Can you work these out from the model? Positions are in its coordinate system, mm. A direction names the side the tool comes from. Give positions to 0.01 mm unless a question says otherwise; leave off trailing zeros. Loops run counter-clockwise (first coordinate to the right, second up) from the corner with the lowest first, then second, coordinate; pieces in that order, holes last. Notation, with made-up numbers: (43.25, 85) -> (62.25, 85) arc R10 cw to (62.25, 101) -> close; hole circle Ø11 at (-28, 78.5). An arc over 180 degrees is marked (long way). One line per question, with ' | ' between items.
from build123d import *

# Parameters (mm, degrees)
F0_W     = 63.2
F0_H     = 30.7
F1_DEPTH = 9
F2_R     = 4.5
F2_R_2   = 3
F3_DEPTH = 3.5
F4_T     = 1


# Not quite as in the source:
# - a shell that OpenCascade refuses in one call is made with other operations: the cavity is built on its own and cut out


with BuildPart() as f1:
    # F0 (on Front) → F1 (new body)
    with BuildSketch(Plane.XZ):
        with Locations((2.7909118284, 0)):
            Rectangle(F0_W, F0_H)
    extrude(amount=F1_DEPTH)

    # F2 (on face) → F3 (join)
    with BuildSketch(Plane.XZ.offset(9)):
        with Locations((-21.0856401334, 7.675)):
            Circle(F2_R)
        with Locations((-21.0856401334, 7.675)):
            Circle(F2_R_2, mode=Mode.SUBTRACT)
        with Locations((-4.9325362097, 7.675)):
            Circle(F2_R)
        with Locations((-4.9325362097, 7.675)):
            Circle(F2_R_2, mode=Mode.SUBTRACT)
        with Locations((10.5143598666, 7.675)):
            Circle(F2_R)
        with Locations((10.5143598666, 7.675)):
            Circle(F2_R_2, mode=Mode.SUBTRACT)
        with Locations((-4.9325362097, -7.675)):
            Circle(F2_R)
        with Locations((-4.9325362097, -7.675)):
            Circle(F2_R_2, mode=Mode.SUBTRACT)
        with Locations((10.5143598666, -7.675)):
            Circle(F2_R)
        with Locations((10.5143598666, -7.675)):
            Circle(F2_R_2, mode=Mode.SUBTRACT)
        with Locations((-21.0856401334, -7.675)):
            Circle(F2_R)
        with Locations((-21.0856401334, -7.675)):
            Circle(F2_R_2, mode=Mode.SUBTRACT)
        with Locations((26.6674637903, -7.675)):
            Circle(F2_R)
        with Locations((26.6674637903, -7.675)):
            Circle(F2_R_2, mode=Mode.SUBTRACT)
        with Locations((26.6674637903, 7.675)):
            Circle(F2_R)
        with Locations((26.6674637903, 7.675)):
            Circle(F2_R_2, mode=Mode.SUBTRACT)
    extrude(amount=F3_DEPTH)

    # F4: shell of thickness 1, made by hand


with BuildPart() as f4_core1:
    # F4_t2: copy of F1
    add(f1.part)

    # the walls: a layer under each face that stays
    f4_faces = [f4_core1.faces().sort_by_distance(p)[0] for p in [
        (2.7909118284, -4.5, -15.35),
        (-28.8090881716, -4.5, 0),
        (34.3909118284, -4.5, 0),
        (2.7909118284, -9, 0),
        (2.7909118284, -4.5, 15.35),
        (-25.5856401334, -10.75, -7.675),
        (-9.4325362097, -10.75, -7.675),
        (6.0143598666, -10.75, -7.675),
        (22.1674637903, -10.75, -7.675),
        (-25.5856401334, -10.75, 7.675),
        (-9.4325362097, -10.75, 7.675),
        (6.0143598666, -10.75, 7.675),
        (22.1674637903, -10.75, 7.675),
        (-24.0856401334, -12.5, -10.675),
        (-7.9325362097, -12.5, -10.675),
        (7.5143598666, -12.5, -10.675),
        (23.6674637903, -12.5, -10.675),
        (-24.0856401334, -12.5, 4.675),
        (-7.9325362097, -12.5, 4.675),
        (7.5143598666, -12.5, 4.675),
        (23.6674637903, -12.5, 4.675),
        (-24.0856401334, -10.75, -7.675),
        (-7.9325362097, -10.75, -7.675),
        (7.5143598666, -10.75, -7.675),
        (23.6674637903, -10.75, -7.675),
        (-24.0856401334, -10.75, 7.675),
        (-7.9325362097, -10.75, 7.675),
        (7.5143598666, -10.75, 7.675),
        (23.6674637903, -10.75, 7.675),
        (-21.0856401334, -9, -7.675),
        (-4.9325362097, -9, -7.675),
        (10.5143598666, -9, -7.675),
        (26.6674637903, -9, -7.675),
        (-21.0856401334, -9, 7.675),
        (-4.9325362097, -9, 7.675),
        (10.5143598666, -9, 7.675),
        (26.6674637903, -9, 7.675),
    ]]
    thicken(f4_faces, amount=-F4_T, mode=Mode.SUBTRACT)

    # F4_s3 → F4_t4 (revolve, cut)
    with BuildSketch(Plane.XY.offset(-7.675)):
        Polygon((-16.5756401334, -9.01), (-16.5856401334, -8), (-17.5856401334, -8), (-17.5856401334, -9), align=None)
    revolve(axis=Axis((-21.0856401334, -9, -7.675), (0, -1, 0)), mode=Mode.SUBTRACT)

    # F4_s5 → F4_t6 (revolve, cut)
    with BuildSketch(Plane.XY.offset(-7.675)):
        Polygon((-0.4225362097, -9.01), (-0.4325362097, -8), (-1.4325362097, -8), (-1.4325362097, -9), align=None)
    revolve(axis=Axis((-4.9325362097, -9, -7.675), (0, -1, 0)), mode=Mode.SUBTRACT)

    # F4_s7 → F4_t8 (revolve, cut)
    with BuildSketch(Plane.XY.offset(-7.675)):
        Polygon((15.0243598666, -9.01), (15.0143598666, -8), (14.0143598666, -8), (14.0143598666, -9), align=None)
    revolve(axis=Axis((10.5143598666, -9, -7.675), (0, -1, 0)), mode=Mode.SUBTRACT)

    # F4_s9 → F4_t10 (revolve, cut)
    with BuildSketch(Plane.XY.offset(-7.675)):
        Polygon((31.1774637903, -9.01), (31.1674637903, -8), (30.1674637903, -8), (30.1674637903, -9), align=None)
    revolve(axis=Axis((26.6674637903, -9, -7.675), (0, -1, 0)), mode=Mode.SUBTRACT)

    # F4_s11 → F4_t12 (revolve, cut)
    with BuildSketch(Plane.XY.offset(7.675)):
        Polygon((-16.5756401334, -9.01), (-16.5856401334, -8), (-17.5856401334, -8), (-17.5856401334, -9), align=None)
    revolve(axis=Axis((-21.0856401334, -9, 7.675), (0, -1, 0)), mode=Mode.SUBTRACT)

    # F4_s13 → F4_t14 (revolve, cut)
    with BuildSketch(Plane.XY.offset(7.675)):
        Polygon((-0.4225362097, -9.01), (-0.4325362097, -8), (-1.4325362097, -8), (-1.4325362097, -9), align=None)
    revolve(axis=Axis((-4.9325362097, -9, 7.675), (0, -1, 0)), mode=Mode.SUBTRACT)

    # F4_s15 → F4_t16 (revolve, cut)
    with BuildSketch(Plane.XY.offset(7.675)):
        Polygon((15.0243598666, -9.01), (15.0143598666, -8), (14.0143598666, -8), (14.0143598666, -9), align=None)
    revolve(axis=Axis((10.5143598666, -9, 7.675), (0, -1, 0)), mode=Mode.SUBTRACT)

    # F4_s17 → F4_t18 (revolve, cut)
    with BuildSketch(Plane.XY.offset(7.675)):
        Polygon((31.1774637903, -9.01), (31.1674637903, -8), (30.1674637903, -8), (30.1674637903, -9), align=None)
    revolve(axis=Axis((26.6674637903, -9, 7.675), (0, -1, 0)), mode=Mode.SUBTRACT)

    # F4_s19 → F4_t20 (revolve, cut)
    with BuildSketch(Plane.XY.offset(-7.675)):
        Polygon((-18.0956401334, -9.01), (-17.0856401334, -9), (-17.0856401334, -8), (-18.0856401334, -8), align=None)
    revolve(axis=Axis((-21.0856401334, -9, -7.675), (0, -1, 0)), mode=Mode.SUBTRACT)

    # F4_s21 → F4_t22 (revolve, cut)
    with BuildSketch(Plane.XY.offset(-7.675)):
        Polygon((-1.9425362097, -9.01), (-0.9325362097, -9), (-0.9325362097, -8), (-1.9325362097, -8), align=None)
    revolve(axis=Axis((-4.9325362097, -9, -7.675), (0, -1, 0)), mode=Mode.SUBTRACT)

    # F4_s23 → F4_t24 (revolve, cut)
    with BuildSketch(Plane.XY.offset(-7.675)):
        Polygon((13.5043598666, -9.01), (14.5143598666, -9), (14.5143598666, -8), (13.5143598666, -8), align=None)
    revolve(axis=Axis((10.5143598666, -9, -7.675), (0, -1, 0)), mode=Mode.SUBTRACT)

    # F4_s25 → F4_t26 (revolve, cut)
    with BuildSketch(Plane.XY.offset(-7.675)):
        Polygon((29.6574637903, -9.01), (30.6674637903, -9), (30.6674637903, -8), (29.6674637903, -8), align=None)
    revolve(axis=Axis((26.6674637903, -9, -7.675), (0, -1, 0)), mode=Mode.SUBTRACT)

    # F4_s27 → F4_t28 (revolve, cut)
    with BuildSketch(Plane.XY.offset(7.675)):
        Polygon((-18.0956401334, -9.01), (-17.0856401334, -9), (-17.0856401334, -8), (-18.0856401334, -8), align=None)
    revolve(axis=Axis((-21.0856401334, -9, 7.675), (0, -1, 0)), mode=Mode.SUBTRACT)

    # F4_s29 → F4_t30 (revolve, cut)
    with BuildSketch(Plane.XY.offset(7.675)):
        Polygon((-1.9425362097, -9.01), (-0.9325362097, -9), (-0.9325362097, -8), (-1.9325362097, -8), align=None)
    revolve(axis=Axis((-4.9325362097, -9, 7.675), (0, -1, 0)), mode=Mode.SUBTRACT)

    # F4_s31 → F4_t32 (revolve, cut)
    with BuildSketch(Plane.XY.offset(7.675)):
        Polygon((13.5043598666, -9.01), (14.5143598666, -9), (14.5143598666, -8), (13.5143598666, -8), align=None)
    revolve(axis=Axis((10.5143598666, -9, 7.675), (0, -1, 0)), mode=Mode.SUBTRACT)

    # F4_s33 → F4_t34 (revolve, cut)
    with BuildSketch(Plane.XY.offset(7.675)):
        Polygon((29.6574637903, -9.01), (30.6674637903, -9), (30.6674637903, -8), (29.6674637903, -8), align=None)
    revolve(axis=Axis((26.6674637903, -9, 7.675), (0, -1, 0)), mode=Mode.SUBTRACT)


with BuildPart() as f1_1:
    add(f1.part)

    # what is left inside the walls is the cavity
    f4_cavity = [f4_core1.part.solids().sort_by_distance(p)[0] for p in [
        (2.790912, -0.01, -4.783333),
    ]]
    add(f4_cavity, mode=Mode.SUBTRACT)


solid = f1_1.part
Q1. For pin 1 Ø3.5 at (x, z) = (-4.93, 7.68) entering from -Y; pin 2 Ø9.5 at (x, z) = (26.67, -7.68) entering from +Y; pin 3 Ø2 at (x, y) = (-12, -10.5) entering from -Z, each with a flat end and sliding along its axis, tell me the tip position at first contact or that it passes through.
Entries:
pin 1: y = -9 | pin 2: y = -8 | pin 3: through
Q2. If we mould it in two halves opening along Z, with no side actions, what happens to faces 1 (the face through (-5.518, -10.726, 12.137)), 2 (the face through (-20, -12.5, -11))? For each: pulls with the +Z half, pulls with the -Z half, needs draft (parallel to the pull), parting line crosses it, or undercut.
Entries:
face 1: undercut | face 2: needs draft
Q3. If we section it at C-C (y = -11): State how many separate pieces and enclosed holes the cut face has, plus the area to 3 significant figures.
Entries:
separate pieces: 8 | enclosed holes: 8 | area: 283 mm²
Q4. If we section it at A-A (y = -5): Write out the boundary of the cut face in (x, z).
Entries:
outline: (-28.81, -15.35) -> (34.39, -15.35) -> (34.39, 15.35) -> (-28.81, 15.35) -> close; hole (-27.81, -14.35) -> (33.39, -14.35) -> (33.39, 14.35) -> (-27.81, 14.35) -> close
Q5. If we section it at D-D (z = -1): Write out the boundary of the cut face in (x, y).
Entries:
outline: (-28.81, -9) -> (34.39, -9) -> (34.39, 0) -> (33.39, 0) -> (33.39, -8) -> (-27.81, -8) -> (-27.81, 0) -> (-28.81, 0) -> close
Q6. If we section it at B-B (x = -14.5): Write out the boundary of the cut face in (y, z), plus the area to 3 significant figures.
Entries:
outline: (-9, -15.35) -> (0, -15.35) -> (0, -14.35) -> (-8, -14.35) -> (-8, 14.35) -> (0, 14.35) -> (0, 15.35) -> (-9, 15.35) -> close | area: 46.7 mm²
Q7. On a 3-axis mill with a long thin cutter (end or side, diameter ignored), from which of +Z, -Z, +X, -X, +Y, -Y can I reach the whole of each face in a straight line? I mean faces 3 (the face through (2, -8, 0)), 4 (the face through (14.807, -10.726, 9.027)), 5 (the face through (-18, -12.5, 7)). Say none if no direction works.
Entries:
face 3: +Y | face 4: -Y | face 5: +Z, -Z, +X, -X, -Y
Q8. If I drill on probe 1 along X at (y, z) = (-2.25, 2); probe 2 along Z at (x, y) = (14.5, -6.5); probe 3 along Y at (x, z) = (-0.5, 0), over which ranges is the centre line in solid material (lowest first)? Write a range as from..to.
Entries:
probe 1: -28.81..-27.81, 33.39..34.39 | probe 2: -15.35..-14.35, 14.35..15.35 | probe 3: -9..-8
